Input: part model. Units: mm. Frame: model coordinates. A direction names the side the tool comes from. Coordinates: 2 decimals unless noted, no trailing zeros. Loops run counter-clockwise (first coordinate to the right, second up) from the corner with the lowest first, then second, coordinate; pieces in that order, holes last.
(1) Line query: L1, parallel to Y at x = -191.1, z = -5; L2, parallel to Y at x = -93.5, z = -166.5; L3, parallel to Y at x = 0, z = -433.5. Output: solid intervals per line, ascending.
(2) Contact query for flat-ended pins moving along their axis: P1, Ø12, axis at x = -124.5, z = -214, coming from the +Y side; P2, Ø4, axis at x = -89.5, y = -182.5, coming from the -Z side; P3, Ø8, axis at x = -48, y = -104, coming from the +Z side. Output: stop coordinate, or through.
(3) Mould query, pull axis X, two halves, no side actions, for faces 6 (the face through (5.5, -24.9, -419.7)), 7 (the face through (-23.846, 7.509, -425.21)), 8 (the face through (-3, 3, -395)), 9 (the face through (-16.9, -18.8, -440)). Classes: released by +X, released by -X, zero draft, split by the parting line, or undercut.
(4) Section D-D, the plane z = -60.5. Return loops of the section in (x, y).
(5) Set-up query: faces 1 (the face through (-8.82, 323.95, -211.51)), 2 (the face through (0, 0, -410)), 3 (the face through (-3, 240, -195)), 4 (the face through (-3, -250, -197)), 5 (the face through (200, -3, -197)). Return all of +Z, -Z, +X, -X, +Y, -Y with unobstructed straight access to the full face (end or side cutting, diameter ignored); none if empty.
(6) Section A-A, the plane z = -200. Return loops of the section in (x, y).
(7) Section B-B, the plane x = 0. Return loops of the section in (y, z).
(8) Section C-C, the plane y = -34. Return loops of the section in (x, z), then the cut area to 3 significant figures.
```python
from build123d import *

# Parameters (mm, degrees)
CROQUIS2_W              = 400
CROQUIS2_H              = 500
SALIENTE_EXTRUIR1_DEPTH = 400
CROQUIS3_W              = 380
CROQUIS3_H              = 480
CORTAR_EXTRUIR1_DEPTH   = 395
CROQUIS4_R              = 25.5
SALIENTE_EXTRUIR4_DEPTH = 40
CROQUIS5_R              = 25
CORTAR_EXTRUIR2_DEPTH   = 30
CROQUIS6_R              = 14.5
SALIENTE_EXTRUIR5_DEPTH = 150
CROQUIS9_R              = 0.75
CORTAR_EXTRUIR4_DEPTH   = 1.5
CORTAR_EXTRUIR5_START   = -1.5
CROQUIS10_R             = 0.75
CORTAR_EXTRUIR5_DEPTH   = 1.5
CROQUIS12_R             = 0.75
CORTAR_EXTRUIR6_DEPTH   = 1.5
CORTAR_EXTRUIR7_START   = -1.5
CROQUIS13_R             = 0.75
CORTAR_EXTRUIR7_DEPTH   = 1.5


with BuildPart() as part:
    # Croquis2 → Saliente-Extruir1 (new body)
    with BuildSketch(Plane.XY):
        Rectangle(CROQUIS2_W, CROQUIS2_H)
    extrude(amount=-SALIENTE_EXTRUIR1_DEPTH)

    # Croquis3 → Cortar-Extruir1 (cut)
    with BuildSketch(Plane.XY):
        Rectangle(CROQUIS3_W, CROQUIS3_H)
    extrude(amount=-CORTAR_EXTRUIR1_DEPTH, mode=Mode.SUBTRACT)

    # Croquis4 → Saliente-Extruir4 (add)
    with BuildSketch(Plane(origin=(0, 0, -400), x_dir=(-1, 0, 0), z_dir=(0, 0, -1))):
        Circle(CROQUIS4_R)
    extrude(amount=SALIENTE_EXTRUIR4_DEPTH)

    # Croquis5 → Cortar-Extruir2 (cut)
    with BuildSketch(Plane(origin=(0, 0, -440), x_dir=(-1, 0, 0), z_dir=(0, 0, -1))):
        Circle(CROQUIS5_R)
    extrude(amount=-CORTAR_EXTRUIR2_DEPTH, mode=Mode.SUBTRACT)

    # Croquis6 → Saliente-Extruir5 (add)
    with BuildSketch(Plane(origin=(0, 250, 0), x_dir=(1, 0, 0), z_dir=(0, 1, 0))):
        with Locations(Location((0, 200, 0), (0, 0, 270))):
            Circle(CROQUIS6_R)
    extrude(amount=SALIENTE_EXTRUIR5_DEPTH)

    # Croquis9 → Cortar-Extruir4 (cut)
    with BuildSketch(Plane.ZY.offset(-190)):
        with Locations((-5, 230)):
            Circle(CROQUIS9_R)
    extrude(amount=-CORTAR_EXTRUIR4_DEPTH, mode=Mode.SUBTRACT)

    # Croquis10 → Cortar-Extruir5 (cut)
    with BuildSketch(Plane(origin=(-190, 0, 0), x_dir=(0, 0, -1), z_dir=(1, 0, 0)).offset(CORTAR_EXTRUIR5_START)):
        with Locations(Location((5, 230, 0), (0, 0, 180))):
            Circle(CROQUIS10_R)
    extrude(amount=CORTAR_EXTRUIR5_DEPTH, mode=Mode.SUBTRACT)

    # Croquis12 → Cortar-Extruir6 (cut)
    with BuildSketch(Plane(origin=(-190, 0, 0), x_dir=(0, 0, -1), z_dir=(1, 0, 0))):
        with Locations((5, -230)):
            Circle(CROQUIS12_R)
    extrude(amount=-CORTAR_EXTRUIR6_DEPTH, mode=Mode.SUBTRACT)

    # Croquis13 → Cortar-Extruir7 (cut)
    with BuildSketch(Plane.ZY.offset(-190).offset(CORTAR_EXTRUIR7_START)):
        with Locations(Location((-5, -230, 0), (0, 0, 180))):
            Circle(CROQUIS13_R)
    extrude(amount=CORTAR_EXTRUIR7_DEPTH, mode=Mode.SUBTRACT)


solid = part.part
```
Report:
1. L1: y = -250 to -230.75, -229.25 to 229.25, 230.75 to 250
1. L2: y = -250 to -240, 240 to 250
1. L3: y = -25.5 to -25, 25 to 25.5
2. P1: stops at y = 250
2. P2: stops at z = -400
2. P3: stops at z = -395
3. face 6: split by the parting line
3. face 7: undercut
3. face 8: undercut
3. face 9: zero draft
4. outline: (-200, -250) - (200, -250) - (200, 250) - (-200, 250) - close; hole (-190, -240) - (190, -240) - (190, 240) - (-190, 240) - close
5. face 1: +Y
5. face 2: -Z
5. face 3: +Z
5. face 4: +Z, -Z, +X, -X, -Y
5. face 5: +Z, -Z, +X, +Y, -Y
6. outline: (-200, -250) - (200, -250) - (200, 250) - (14.5, 250) - (14.5, 400) - (-14.5, 400) - (-14.5, 250) - (-200, 250) - close; hole (-190, -240) - (190, -240) - (190, 240) - (-190, 240) - close
7. outline: (-250, -400) - (-25.5, -400) - (-25.5, -440) - (-25, -440) - (-25, -410) - (25, -410) - (25, -440) - (25.5, -440) - (25.5, -400) - (250, -400) - (250, -214.5) - (400, -214.5) - (400, -185.5) - (250, -185.5) - (250, 0) - (240, 0) - (240, -395) - (-240, -395) - (-240, 0) - (-250, 0) - close
8. outline: (-200, -400) - (200, -400) - (200, 0) - (190, 0) - (190, -395) - (-190, -395) - (-190, 0) - (-200, 0) - close
8. area: 9,900 mm2
